Part model, mm, in its own coordinate system. A direction names the side the tool comes from. Round coordinates to 2 decimals unless told otherwise and drop trailing zeros. Loops run counter-clockwise (first coordinate to the right, second up) from the corner with the lowest first, then second, coordinate; pieces in that order, holes last.
(1) Tool access for faces 1 (the face through (50, -1, 14)), 2 (the face through (-51.014, -34.075, 18.686)): list every direction of +Z, -Z, +X, -X, +Y, -Y with a clear straight run to the whole face (end or side of a thin tool).
(2) Probe probe 1 along X at (y, z) = (27, 13); probe 2 along Z at (x, y) = (50.95, 1); probe 3 along Z at (x, y) = (35.5, 21.5). List the from-to ranges inside material, lowest first.
(3) Cut at D-D on x = 0. List the corners of the cut face in (y, z).
(4) Mould opens along Y. For faces 3 (the face through (-51, 1, 19)), 4 (the face through (-16, -52, 1)), 5 (the face through (-52, -1, 13)) say: +Y half, -Y half, draft (parallel to the pull), parting line (faces both ways), or undercut.
(5) Cut at A-A on z = 17. Count the separate pieces of the cut face and the enclosed holes in it, then the cut area to 3 significant figures.
(6) Flat gauge pin, fed straight in: pin 1 (4 mm diameter, centred on x = -22.5, y = 33.5, fed in from +Z). Where does the tip first touch, or does it go through?
from build123d import *

# Parameters (mm, degrees)
F0_W     = 104
F0_H     = 104
F1_DEPTH = 2
F2_W     = 2
F2_H     = 104
F3_DEPTH = 25
F4_W     = 2
F4_H     = 104
F5_DEPTH = 25
F6_R     = 0.99999
F7_R     = 0.99999
F9_D     = 4
F11_D    = 4
F13_D    = 4


# Not quite as in the source:
# - a fillet or chamfer is up to 0.001 mm smaller than in the source, because OpenCascade refuses the exact size


with BuildPart() as f1:
    # F0 (on Top) → F1 (new body)
    with BuildSketch(Plane.XY):
        Rectangle(F0_W, F0_H)
    extrude(amount=F1_DEPTH)

    # F2 (on face) → F3 (join)
    with BuildSketch(Plane.XY.offset(2)):
        with Locations((-51, 0)):
            Rectangle(F2_W, F2_H)
    extrude(amount=F3_DEPTH)

    # F4 (on face) → F5 (join)
    with BuildSketch(Plane.XY.offset(2)):
        with Locations((51, 0)):
            Rectangle(F4_W, F4_H)
    extrude(amount=F5_DEPTH)

    # F6 (radius 1 in the source; OpenCascade refuses exactly that, so slightly less here)
    f6_edges = [f1.edges().sort_by_distance(p)[0] for p in [
        (52, 0, 27),
        (51, 52, 27),
        (50, 0, 27),
        (51, -52, 27),
    ]]
    fillet(f6_edges, radius=F6_R)

    # F7 (radius 1 in the source; OpenCascade refuses exactly that, so slightly less here)
    f7_edges = [f1.edges().sort_by_distance(p)[0] for p in [
        (-51, 52, 27),
        (-52, 0, 27),
        (-51, -52, 27),
        (-50, 0, 27),
    ]]
    fillet(f7_edges, radius=F7_R)

    # F9 (through all)
    with Locations(Plane.YZ.offset(52)):
        with Locations((-33, 17)):
            Hole(F9_D / 2)

    # F11 (through all)
    with Locations(Plane.YZ.offset(52)):
        with Locations((1, 17)):
            Hole(F11_D / 2)

    # F13 (through all)
    with Locations(Plane.YZ.offset(52)):
        with Locations((35, 17)):
            Hole(F13_D / 2)


solid = f1.part
Final values:
1. face 1: +Z, +Y, -Y
1. face 2: +X, -X
2. probe 1: x = -52 to -50, 50 to 52
2. probe 2: z = 0 to 15, 19 to 27
2. probe 3: z = 0 to 2
3. outline: (-52, 0) - (52, 0) - (52, 2) - (-52, 2) - close
4. face 3: undercut
4. face 4: -Y half
4. face 5: draft
5. separate pieces: 8
5. enclosed holes: 0
5. area: 368 mm2
6. pin 1: stops at z = 2
